from build123d import *

# Parameters (mm, degrees)
F1_DEPTH = 11.1125


# Not quite as in the source:
# - a length typed as a fraction of an inch, garbled in the dataset ("3 / 203.2 mm" for 3/8 in), is restored


with BuildPart() as f1:
    # F0 (on Top) → F1 (new body)
    with BuildSketch(Plane.XY):
        with BuildLine():
            ThreePointArc((-0.1411418198, 20.1985444874), (-5.0054503986, 18.2564119782), (-9.2097157612, 15.1327075437))
            ThreePointArc((-9.2097157612, 15.1327075437), (-10.6205392688, 11.8246856933), (-10.2093555033, 8.2519613206))
            Line((-10.2093555033, 8.2519613206), (-12.369341217, 7.1464567445))
            Line((-12.369341217, 7.1464567445), (-12.369341217, 4.6386048198))
            Line((-12.369341217, 4.6386048198), (-12.369341217, 4.5682978211))
            ThreePointArc((-12.369341217, 4.5682978211), (-15.5930977879, 3.1185654947), (-17.7027139134, 0.2823972963))
            ThreePointArc((-17.7027139134, 0.2823972963), (-18.3641606661, -4.889059653), (-17.5542831421, -10.0393583998))
            ThreePointArc((-17.5542831421, -10.0393583998), (-13.4613837791, -13.3941238354), (-8.5996589687, -15.484556372))
            ThreePointArc((-8.5996589687, -15.484556372), (-5.0294162563, -15.0523544446), (-2.1409380715, -12.9098966718))
            Line((-2.1409380715, -12.9098966718), (0, -14.2561570176))
            Line((0, -14.2561570176), (1.9696742658, -12.9098966718))
            ThreePointArc((1.9696742658, -12.9098966718), (4.9392756736, -15.0084468105), (8.560301624, -15.3410370587))
            ThreePointArc((8.560301624, -15.3410370587), (13.367982191, -13.3015402533), (17.4874793738, -10.0916987285))
            ThreePointArc((17.4874793738, -10.0916987285), (18.16772005, -4.8427956267), (17.6633565687, 0.4259166096))
            ThreePointArc((17.6633565687, 0.4259166096), (15.4847616458, 3.3168082822), (12.1560195839, 4.739132713))
            Line((12.1560195839, 4.739132713), (12.1560195839, 7.1464567445))
            Line((12.1560195839, 7.1464567445), (9.9960338703, 8.2519613206))
            ThreePointArc((9.9960338703, 8.2519613206), (10.4072176357, 11.8246856933), (8.9963941282, 15.1327075437))
            ThreePointArc((8.9963941282, 15.1327075437), (4.7823081966, 18.3053860292), (-0.1411418198, 20.1985444874))
        make_face()
    extrude(amount=F1_DEPTH)


solid = f1.part
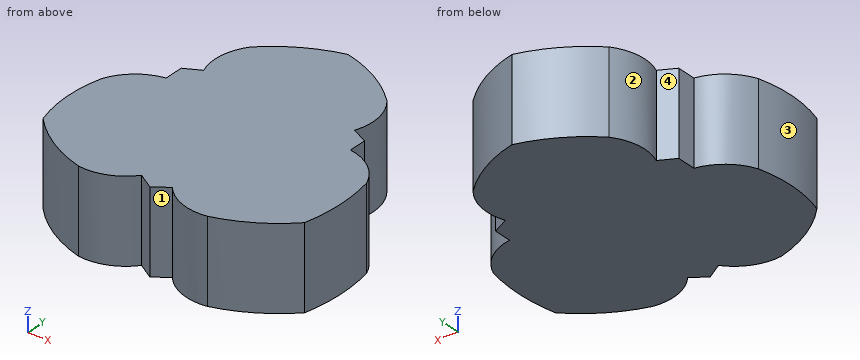
The listing builds one solid part. Answer for the finished solid, in the listing's coordinates (mm). Face numbers are marked on the shaded views. Round coordinates to 2 decimals unless told otherwise and drop trailing zeros. Order: outer loops, then holes, each group sorted by start corner. A loop starts at its lowest first (then second) coordinate and runs counter-clockwise, first axis right, second up. Notation, with made-up numbers: (58.5, 78) -> (82.5, 78) arc R23 cw to (82.5, 96) -> close; hole circle Ø6 at (36.25, 29). An arc over 180 degrees is marked (long way). Write each question's results on one line, items separated by ' | '. Start each with the question number.
Q1. The mould has two halves that part along Y. Classify the marked faces 1, 2, 3 and 4: pulls with the +Y half, pulls with the -Y half, needs draft (parallel to the pull), parting line crosses it, or undercut.
Q2. Each of these flat-tipped pins is pushed along its axis until it touches: pin 1 (3 mm diameter, centred on y = 11, z = 5.5, fed in from +X); pin 2 (6 mm diameter, centred on x = -1.5, y = 13, fed in from -Z); pin 3 (0.8 mm diameter, centred on y = 6.5, z = 7, fed in from -X); pin 4 (2 mm diameter, centred on y = 2.5, z = 1.5, fed in from -X). Where does it stop, or does it pass through?
Q3. Find section B-B (x = 11). Determine the outline of the cut face in (y, z), then the cut area to 3 significant figures.
Q4. Find section C-C (y = 10). Determine the outline of the cut face in (x, z), then the cut area to 3 significant figures.
Q5. Straight lines are drawn through the part: probe 1 along X at (y, z) = (11, 6.5); probe 2 along X at (y, z) = (5, 5.25); probe 3 along Y at (x, z) = (-4, 9.25). For each, find the intervals that lie inside material, in ascending order. Write a range as from..to.
Q6. Find section A-A (z = 3.75). Determine the outline of the cut face in (x, y).
Worked answers:
1) face 1: pulls with the -Y half | face 2: undercut | face 3: parting line crosses it | face 4: undercut
2) pin 1: stops at x = 10.48 | pin 2: stops at z = 0 | pin 3: stops at x = -12.37 | pin 4: stops at x = -17.06
3) outline: (-14.49, 0) -> (7.74, 0) -> (7.74, 11.11) -> (-14.49, 11.11) -> close | area: 247 mm2
4) outline: (-10.65, 0) -> (10.43, 0) -> (10.43, 11.11) -> (-10.65, 11.11) -> close | area: 234 mm2
5) probe 1: x = -10.69..10.48 | probe 2: x = -12.37..12.16 | probe 3: y = -14.54..18.78
6) outline: (-17.7, 0.28) arc R18.47 ccw to (-17.55, -10.04) arc R18.93 ccw to (-8.6, -15.48) arc R7.02 ccw to (-2.14, -12.91) -> (0, -14.26) -> (1.97, -12.91) arc R7.02 ccw to (8.56, -15.34) arc R20.09 ccw to (17.49, -10.09) arc R23.64 ccw to (17.66, 0.43) arc R7.02 ccw to (12.16, 4.74) -> (12.16, 7.15) -> (10, 8.25) arc R7.02 ccw to (9, 15.13) arc R19.02 ccw to (-0.14, 20.2) arc R20.27 ccw to (-9.21, 15.13) arc R7.02 ccw to (-10.21, 8.25) -> (-12.37, 7.15) -> (-12.37, 4.57) arc R7.02 ccw to start
